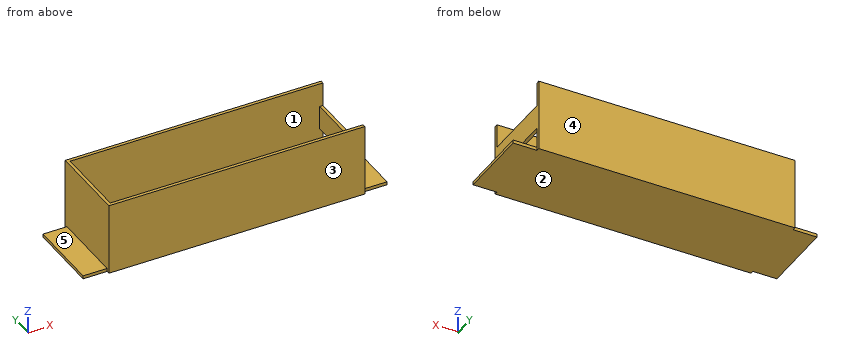
```python
from build123d import *

# Parameters (mm, degrees)
ESBO_O1_W                = 160
ESBO_O1_H                = 50
RESSALTO_EXTRUS_O1_DEPTH = 45
ESBO_O3_W                = 2
ESBO_O3_H                = 46
RESSALTO_EXTRUS_O2_DEPTH = 15
ESBO_O9_W                = 156
ESBO_O9_H                = 46
CORTE_EXTRUS_O2_DEPTH    = 43
CORTE_EXTRUS_O3_REACH    = 162
ESBO_O10_W               = 15
ESBO_O10_H               = 46
ESBO_O10_W_2             = 13
ESBO_O11_W               = 2
ESBO_O11_H               = 46
RESSALTO_EXTRUS_O6_DEPTH = 15


with BuildPart() as part:
    # Esboço1 → Ressalto-extrusão1 (new body)
    with BuildSketch(Plane.XY):
        Rectangle(ESBO_O1_W, ESBO_O1_H)
    extrude(amount=RESSALTO_EXTRUS_O1_DEPTH)

    # Esboço3 → Ressalto-extrusão2 (add)
    with BuildSketch(Plane(origin=(80, 0, 0), x_dir=(0, 0, -1), z_dir=(1, 0, 0))):
        with Locations((-1, 0)):
            Rectangle(ESBO_O3_W, ESBO_O3_H)
    extrude(amount=RESSALTO_EXTRUS_O2_DEPTH)

    # Esboço9 → Corte-extrusão2 (cut)
    with BuildSketch(Plane.XY.offset(45)):
        Rectangle(ESBO_O9_W, ESBO_O9_H)
    extrude(amount=-CORTE_EXTRUS_O2_DEPTH, mode=Mode.SUBTRACT)

    # Esboço10 → Corte-extrusão3 (cut, up to next)
    with BuildSketch(Plane(origin=(80, 0, 0), x_dir=(0, 0, -1), z_dir=(1, 0, 0)), mode=Mode.PRIVATE) as corte_extrus_o3_sk1:
        with Locations((-37.5, 0)):
            Rectangle(ESBO_O10_W, ESBO_O10_H)
    corte_extrus_o3_tool1 = extrude(corte_extrus_o3_sk1.sketch, amount=-CORTE_EXTRUS_O3_REACH, mode=Mode.PRIVATE) & part.part
    add(corte_extrus_o3_tool1.solids().sort_by_distance((80, 0, 37.5))[0], mode=Mode.SUBTRACT)
    # Esboço10 → Corte-extrusão3 (cut, up to next)
    with BuildSketch(Plane(origin=(80, 0, 0), x_dir=(0, 0, -1), z_dir=(1, 0, 0)), mode=Mode.PRIVATE) as corte_extrus_o3_sk2:
        with Locations((-8.5, 0)):
            Rectangle(ESBO_O10_W_2, ESBO_O10_H)
    corte_extrus_o3_tool2 = extrude(corte_extrus_o3_sk2.sketch, amount=-CORTE_EXTRUS_O3_REACH, mode=Mode.PRIVATE) & part.part
    add(corte_extrus_o3_tool2.solids().sort_by_distance((80, 0, 8.5))[0], mode=Mode.SUBTRACT)

    # Esboço11 → Ressalto-extrusão6 (add)
    with BuildSketch(Plane.ZY.offset(80)):
        with Locations((1, 0)):
            Rectangle(ESBO_O11_W, ESBO_O11_H)
    extrude(amount=RESSALTO_EXTRUS_O6_DEPTH)


solid = part.part
```
Check sheet for the modelled part. Datum: model origin and axes. Units: mm. Face numbers are marked on the shaded views. A direction names the side the tool comes from. Coordinates: 2 decimals unless noted, no trailing zeros. Order: outer loops, then holes, each group sorted by start corner. A loop starts at its lowest first (then second) coordinate and runs counter-clockwise, first axis right, second up. Notation, with made-up numbers: M -3.75,43.25 L 38.25,43.25 A20 ccw 38.25,78.25 Z; hole C 49,27.25 d8. An arc over 180 degrees is marked long. Write each question's results on one line, items separated by ' | '. Start each with the question number.
1. Access from +Z, -Z, +X, -X, +Y, -Y to the whole of each face (thin tool, end or side, straight path). Record for the marked faces 4 and 5.
2. Material ranges on probe 1 along Y at (x, z) = (-69.5, 13.5); probe 2 along X at (y, z) = (-8.5, 17); probe 3 along Z at (x, y) = (4.5, -6), recorded low to high.
3. Cross-section at D-D on x = -36.5. Record the cut outline in (y, z), and give its area (3 significant figures).
4. Cross-section at A-A on y = -3.5. Record the cut outline in (x, z), and give its area (3 significant figures).
5. Go/stop test with flat-tipped pins: P1, Ø4, axis at y = 11.5, z = 16.5, coming from the -X side; P2, Ø6, axis at y = 3.5, z = 19, coming from the +X side; P3, Ø2, axis at x = -90.5, z = 0.5, coming from the -Y side. Record where each tip stops, or that it passes through.
6. Mould release check, pull along Y, two halves, no side actions. Record for the marked faces 1, 2 and 3: +Y half, -Y half, draft (parallel to the pull), parting line (faces both ways), or undercut.
7. Cross-section at B-B on z = 22. Record the cut outline in (x, y), and give its area (3 significant figures).
8. Cross-section at C-C on z = 35. Record the cut outline in (x, y), and give its area (3 significant figures).
Checks:
1) face 4: +Z, -Z, +X, -X, +Y | face 5: +Z, -X, +Y, -Y
2) probe 1: y = -25 to -23, 23 to 25 | probe 2: x = -80 to -78, 78 to 80 | probe 3: z = 0 to 2
3) outline: M -25,0 L 25,0 L 25,45 L 23,45 L 23,2 L -23,2 L -23,45 L -25,45 Z | area: 272 mm²
4) outline: M -95,0 L 95,0 L 95,2 L -78,2 L -78,45 L -80,45 L -80,2 L -95,2 Z; M 78,15 L 80,15 L 80,30 L 78,30 Z | area: 496 mm²
5) P1: stops at x = -80 | P2: stops at x = 80 | P3: stops at y = -23
6) face 1: undercut | face 2: draft | face 3: -Y half
7) outline: M -80,-25 L 80,-25 L 80,25 L -80,25 Z; hole M -78,-23 L 78,-23 L 78,23 L -78,23 Z | area: 824 mm²
8) outline: M -80,-25 L 80,-25 L 80,-23 L -78,-23 L -78,23 L 80,23 L 80,25 L -80,25 Z | area: 732 mm²
